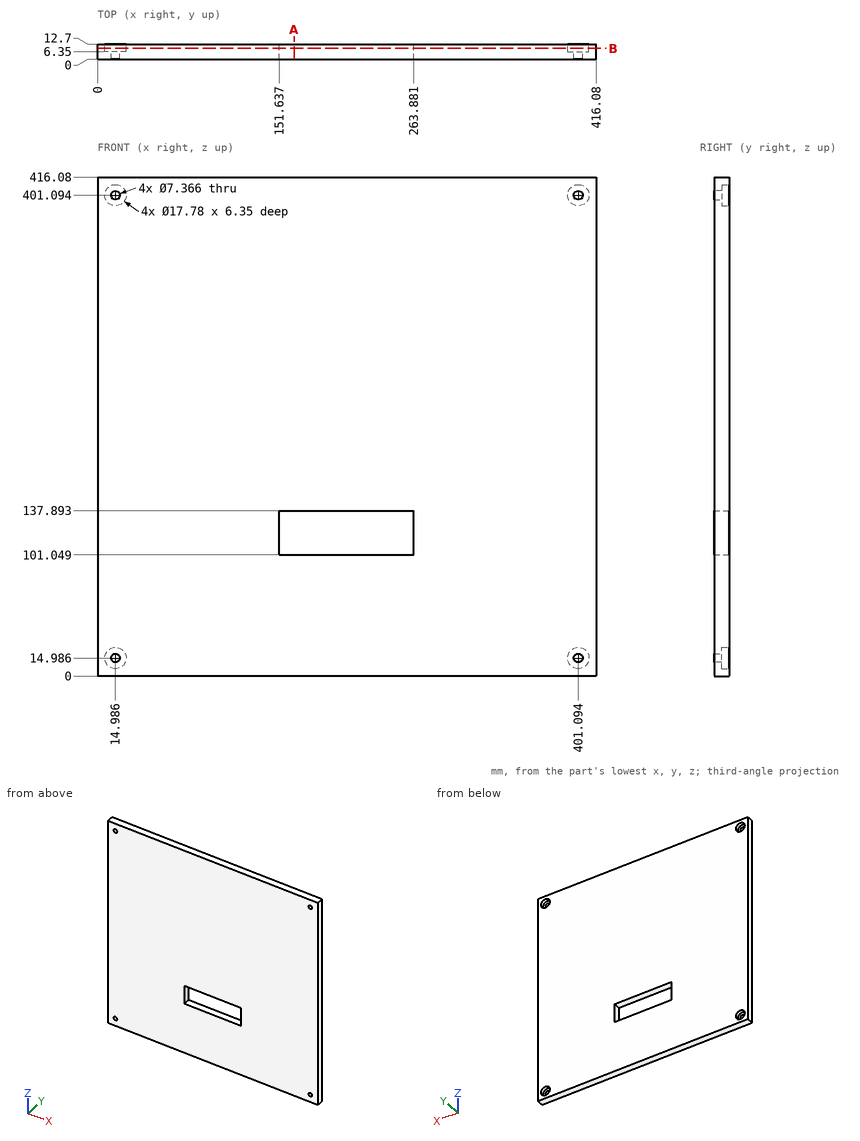
Part print with two shaded views. Sizes in mm from the minimum x, y, z corner. Give positions to 0.01 mm unless a question says otherwise; leave off trailing zeros. Loops run counter-clockwise (first coordinate to the right, second up) from the corner with the lowest first, then second, coordinate; pieces in that order, holes last. Notation, with made-up numbers: (58, 1.25) -> (86, 1.25) arc R11 cw to (86, 11.25) -> close; hole circle Ø8 at (70.5, 85). An arc over 180 degrees is marked (long way). One line per question, with ' | ' between items.
Q1. Cut at A-A, the plane x = 164. Write the cut outline in (y, z), plus the area to 3 significant figures.
Filled sheet:
outline: (0, 0) -> (12.7, 0) -> (12.7, 101.05) -> (0, 101.05) -> close; (0, 137.89) -> (12.7, 137.89) -> (12.7, 416.08) -> (0, 416.08) -> close | area: 4,820 mm²
Q2. Drill centre lines: line 1 along Z through (x, y) = (152, 1.25); line 2 along X through (y, z) = (6.25, 129). Where is each one in solid material? Low to high. Write a range as [from, to].
Filled sheet:
line 1: z = [0, 101.05], [137.89, 416.08] | line 2: x = [0, 151.64], [263.88, 416.08]
Q3. Cut at B-B, the plane y = 9. Write the cut outline in (x, z).
Filled sheet:
outline: (0, 0) -> (416.08, 0) -> (416.08, 416.08) -> (0, 416.08) -> close; hole circle Ø17.78 at (14.99, 14.99); hole circle Ø17.78 at (14.99, 401.09); hole (151.64, 101.05) -> (263.88, 101.05) -> (263.88, 137.89) -> (151.64, 137.89) -> close; hole circle Ø17.78 at (401.09, 14.99); hole circle Ø17.78 at (401.09, 401.09)
Q4. Drop flat-ended pins along their axis: pin 1 (14 mm diameter, centred on x = 12, z = 17, fed in from +Y); pin 2 (16 mm diameter, centred on x = 14.986, z = 14.986, fed in from +Y). Give the stop position or say it passes through.
Filled sheet:
pin 1: stops at y = 12.7 | pin 2: stops at y = 6.35
